Geometry check sheet. Reference: the model listing, model coordinates, mm. Give positions to 0.01 mm unless a question says otherwise; leave off trailing zeros. Order: outer loops, then holes, each group sorted by start corner. A loop starts at its lowest first (then second) coordinate and runs counter-clockwise, first axis right, second up. Notation, with made-up numbers: M 19,11 L 56,11 A33 cw 56,45 Z; hole C 24,5.25 d5. An arc over 180 degrees is marked long. Answer as CSV lines item,"result". Start each with the question number.
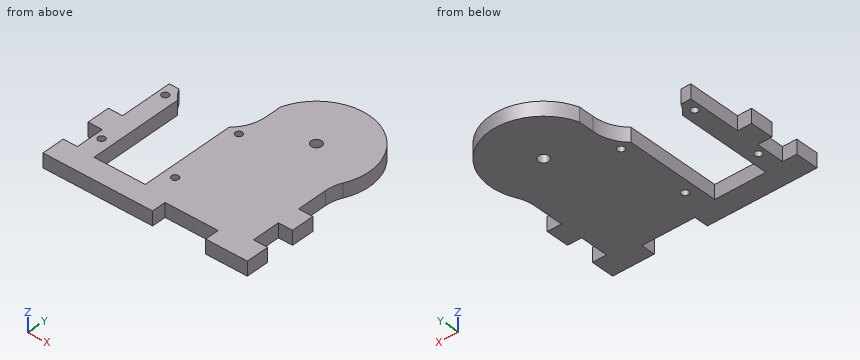
```python
from build123d import *

# Parameters (mm, degrees)
SKETCH_1_R          = 1
SKETCH_1_R_2        = 1.5
EXTRUDE_1_DEPTH     = 4
SKETCH_2_W          = 15
SKETCH_2_H          = 4
CUT_EXTRUDE_1_DEPTH = 10
SKETCH_3_W          = 4
SKETCH_3_H          = 6.5
EXTRUDE_2_DEPTH     = 4


with BuildPart() as part:
    # Эскиз1 → Бобышка-Вытянуть1 (new body)
    with BuildSketch(Plane.XY):
        with BuildLine():
            Line((0, 0), (0, 30))
            Line((0, 30), (2.783140074, 30))
            ThreePointArc((2.783140074, 30), (3.822293637, 28.324390962), (5.15, 26.866755347))
            Line((5.15, 26.866755347), (5.15, 0))
            Line((5.15, 0), (19.65, 0))
            Line((19.65, 0), (19.65, 26.866755347))
            ThreePointArc((19.65, 26.866755347), (22.29801609, 30.609753984), (23.145479479, 35.115731548))
            Line((23.145479479, 35.115731548), (23.145479479, 39.473981947))
            ThreePointArc((23.145479479, 39.473981947), (43.080010933, 48.687001602), (50.84, 28.143198519))
            ThreePointArc((50.84, 28.143198519), (50.063470844, 25.983008862), (49.8, 23.702658011))
            Line((49.8, 23.702658011), (49.8, -6))
            Line((49.8, -6), (0, -6))
            Line((0, -6), (0, 0))
        make_face()
        with Locations((2, 26.5)):
            Circle(SKETCH_1_R, mode=Mode.SUBTRACT)
        with Locations(Location((22.8, 26.5, 0), (0, 0, 180))):
            Circle(SKETCH_1_R, mode=Mode.SUBTRACT)
        with Locations((22.8, 6)):
            Circle(SKETCH_1_R, mode=Mode.SUBTRACT)
        with Locations(Location((2, 6, 0), (0, 0, 180))):
            Circle(SKETCH_1_R, mode=Mode.SUBTRACT)
        with Locations((37.4, 34.80400928)):
            Circle(SKETCH_1_R_2, mode=Mode.SUBTRACT)
    extrude(amount=EXTRUDE_1_DEPTH)

    # Эскиз2 → Вырез-Вытянуть1 (cut)
    with BuildSketch(Plane.XY.offset(4)):
        with Locations((34.5, -4)):
            Rectangle(SKETCH_2_W, SKETCH_2_H)
    extrude(amount=-CUT_EXTRUDE_1_DEPTH, mode=Mode.SUBTRACT)

    # Эскиз3 → Бобышка-Вытянуть2 (add)
    with BuildSketch(Plane.XY.offset(4)):
        with Locations((-2, -2.75)):
            Rectangle(SKETCH_3_W, SKETCH_3_H)
        with Locations((-2, 11.75)):
            Rectangle(SKETCH_3_W, SKETCH_3_H)
        with Locations((51.8, 11.75)):
            Rectangle(SKETCH_3_W, SKETCH_3_H)
        with Locations((51.8, -2.75)):
            Rectangle(SKETCH_3_W, SKETCH_3_H)
    extrude(amount=-EXTRUDE_2_DEPTH)


solid = part.part
```
Item 1: Section check A-A on x = 2. Record the boundary of the cut face in (y, z).
Item 2: Section check D-D on z = 3.05. Give the number of separate pieces and of enclosed holes in the cut face, then the cut area to 3 significant figures.
Item 3: Scan lines: line 1 along Y through (x, z) = (2, 0.9); line 2 along X through (y, z) = (21, 3.45); line 3 along X through (y, z) = (13, 3.8). Record each from-to range of solid material in increasing order.
Item 4: Section check B-B on x = 37.4. Record the boundary of the cut face in (y, z), then the cut area to 3 significant figures.
Item 5: Depth check by flat-ended pin: pin 1 Ø1.4 at (x, z) = (1.5, 2) entering from +Y; pin 2 Ø1 at (y, z) = (25.5, 3) entering from -X; pin 3 Ø1.2 at (x, y) = (22.8, 26.5) entering from -Z; pin 4 Ø2 at (x, z) = (-1.5, 2) entering from +Y. Enter the tip coordinate at first touch or a pass-through.
Item 6: Section check C-C on y = 20.5. Record the boundary of the cut face in (x, z).
Numbers:
1,outline,"M -6,0 L 5,0 L 5,4 L -6,4 Z; M 7,0 L 25.5,0 L 25.5,4 L 7,4 Z; M 27.5,0 L 30,0 L 30,4 L 27.5,4 Z"
2,separate pieces,"1"
2,enclosed holes,"5"
2,area,"1,870 mm2"
3,line 1,"-6 to 5, 7 to 25.5, 27.5 to 30"
3,line 2,"0 to 5.15, 19.65 to 49.8"
3,line 3,"-4 to 5.15, 19.65 to 53.8"
4,outline,"M -2,0 L 33.3,0 L 33.3,4 L -2,4 Z; M 36.3,0 L 49.8,0 L 49.8,4 L 36.3,4 Z"
4,area,"195 mm2"
5,pin 1,"y = 30"
5,pin 2,"x = 0"
5,pin 3,"through"
5,pin 4,"y = 15"
6,outline,"M 0,0 L 5.15,0 L 5.15,4 L 0,4 Z; M 19.65,0 L 49.8,0 L 49.8,4 L 19.65,4 Z"
